```python
from build123d import *

# Parameters (mm, degrees)
F0_W     = 25.4
F0_H     = 12.7
F1_DEPTH = 15.24
F2_R     = 12.7
F3_DEPTH = 12.7
F4_R     = 8.255
F5_DEPTH = 25.4
F7_DEPTH = 3.81


with BuildPart() as f1:
    # F0 (on Top) → F1 (new body)
    with BuildSketch(Plane.XY):
        Rectangle(F0_W, F0_H)
    extrude(amount=F1_DEPTH)

    # F2 (on face) → F3 (join)
    with BuildSketch(Plane.XZ.offset(6.35)):
        Circle(F2_R)
    extrude(amount=-F3_DEPTH)

    # F4 (on face) → F5 (cut)
    with BuildSketch(Plane.XZ.offset(6.35)):
        Circle(F4_R)
    extrude(amount=-F5_DEPTH, mode=Mode.SUBTRACT)

    # F6 (on face) → F7 (join)
    with BuildSketch(Plane.XY.offset(15.24)):
        Polygon((15.698063, -5.10061), (9.701937, 13.35357), (-9.701937, 13.35357), (-15.698063, -5.10061), (0, -16.505921), align=None)
    extrude(amount=F7_DEPTH)


solid = f1.part
```
The model under review builds one solid part; all positions refer to its coordinate system, in mm. A direction names the side the tool comes from. Give positions to 0.01 mm unless a question says otherwise; leave off trailing zeros. Write each loop counter-clockwise with the first axis right and the second up, starting at its lowest first coordinate (ties: lowest second). Pieces come first, ordered by that corner, then holes. Notation, with made-up numbers: M -4.75,-10 L 2.25,-10 A18 cw 2.25,13 Z; hole C -23,-11 d9. An arc over 180 degrees is marked long. Write item = value, one per line. Start each with the question number.
Q1. Clearance check with flat-ended pins moving along their axes: pin 1 (3 mm diameter, centred on x = -5.5, z = -8, fed in from -Y); pin 2 (10 mm diameter, centred on x = 7, y = -5, fed in from -Z); pin 3 (6 mm diameter, centred on x = -12.5, z = 15.5, fed in from -Y); pin 4 (15 mm diameter, centred on x = 0, z = 0, fed in from -Y). State where each tip first meets the part, or that it passes through.
Q2. Mouldability with a two-part tool opening along Z and no side actions: class faces 5 (the face through (12.7, 0, 8)), 6 (the face through (7.874, -0.089, 2.48)), 7 (the face through (-0.279, -0.089, -12.697)) as released by +Z, released by -Z, zero draft, split by the parting line, or undercut.
Q3. Machinability: for faces 1 (the face through (5, -6.35, 7)), 2 (the face through (-12.7, 0, 8)), 3 (the face through (-12.658, 4.256, 17.118)), 4 (the face through (0, 10, 15.24)), which of the approach directions +Z, -Z, +X, -X, +Y, -Y give a long, thin tool a straight path to every point of the face, cutting with its end or side? Answer none if there is none.
Q4. We need section A-A (x = -7). State the section outline as (y, z) points.
Q5. We need section C-C (y = 5.5). State the section outline as (x, z) points (3 decimals), plus the area to 3 significant figures.
Q6. We need section D-D (x = 1). State the section outline as (y, z) points.
Q7. We need section B-B (z = -7.5). State the section outline as (x, y) points, plus the area to 3 significant figures.
Q8. For line 1 (Z direction, x = 0, y = 3.5) (3 decimals); line 2 (Z direction, x = 3, y = -9.75); line 3 (Y direction, x = 11.5, z = 7), list the stretches that pass through material, from the lowest coordinate up.
Result set:
q1.pin_1 = -6.35
q1.pin_2 = -12.54
q1.pin_3 = -9.6
q1.pin_4 = through
q2.face_5 = zero draft
q2.face_6 = undercut
q2.face_7 = released by -Z
q3.face_1 = -Z, +X, -X, -Y
q3.face_2 = -Z, -X, +Y, -Y
q3.face_3 = +Z, -X, +Y
q3.face_4 = -Z, +X, -X, +Y
q4.outline = M -11.42,15.24 L -6.35,15.24 L -6.35,4.38 L 6.35,4.38 L 6.35,15.24 L 13.35,15.24 L 13.35,19.05 L -11.42,19.05 Z; M -6.35,-10.6 L 6.35,-10.6 L 6.35,-4.38 L -6.35,-4.38 Z
q5.outline = M -12.7,0 A12.7 ccw 12.7,0 L 12.7,15.24 L 12.254,15.24 L 12.254,19.05 L -12.254,19.05 L -12.254,15.24 L -12.7,15.24 Z; hole C 0,0 d16.51
q5.area = 520 mm2
q6.outline = M -15.78,15.24 L -6.35,15.24 L -6.35,8.19 L 6.35,8.19 L 6.35,15.24 L 13.35,15.24 L 13.35,19.05 L -15.78,19.05 Z; M -6.35,-12.66 L 6.35,-12.66 L 6.35,-8.19 L -6.35,-8.19 Z
q7.outline = M -10.25,-6.35 L -3.45,-6.35 L -3.45,6.35 L -10.25,6.35 Z; M 3.45,-6.35 L 10.25,-6.35 L 10.25,6.35 L 3.45,6.35 Z
q7.area = 173 mm2
q8.line_1 = -12.7 to -8.255, 8.255 to 19.05
q8.line_2 = 15.24 to 19.05
q8.line_3 = -6.35 to 6.35
